Check sheet for the modelled part. Datum: model origin and axes. Units: mm. Round coordinates to 2 decimals unless told otherwise and drop trailing zeros. Write each loop counter-clockwise with the first axis right and the second up, starting at its lowest first coordinate (ties: lowest second). Pieces come first, ordered by that corner, then holes. Notation, with made-up numbers: (-25, -26.75) -> (-13, -26.75) arc R13 cw to (-13, -4.75) -> close; hole circle Ø5 at (53.25, 78.25). An arc over 180 degrees is marked (long way). Write item = value, one per line.
Solid Edge part; units mm, degrees
sketch "Sketch1" plane through (0, 0, 0) normal (0, 0, 1) x (1, 0, 0)
  line L0 (-36.25, 27.5) -> (36.25, 27.5)
  line L1 (36.25, 27.5) -> (36.25, -27.5)
  line L2 (36.25, -27.5) -> (-36.25, -27.5)
  line L3 (-36.25, -27.5) -> (-36.25, 27.5)
extrude "ExtrudedProtrusion_7" add sketch "Sketch1" along normal blind 4.8
sketch "Sketch2" plane through (0, 0, 4.8) normal (0, 0, 1) x (1, 0, 0)
  line L0 (-33.85, -15) -> (-31.45, -15)
  line L1 (-31.45, -11.9) -> (-31.45, 11.9)
  line L2 (-33.85, 15) -> (-31.45, 15)
  line L3 (-33.85, 15) -> (-33.85, -15)
  arc A0 (-31.45, -11.9) -> (-31.45, -15) centre (-31.45, -13.45) cw
  arc A1 (-31.45, 15) -> (-31.45, 11.9) centre (-31.45, 13.45) cw
  line L4 (31.45, -15) -> (33.85, -15)
  line L5 (33.85, -15) -> (33.85, 15)
  line L6 (33.85, 15) -> (31.45, 15)
  line L7 (31.45, 11.9) -> (31.45, -11.9)
  arc A2 (31.45, 11.9) -> (31.45, 15) centre (31.45, 13.45) cw
  arc A3 (31.45, -15) -> (31.45, -11.9) centre (31.45, -13.45) cw
extrude "ExtrudedCutout_13" cut sketch "Sketch2" against normal blind 2.4
sketch "Sketch3" plane through (0, 0, 4.8) normal (0, 0, 1) x (1, 0, 0)
  line L0 (-33.85, 11.9) -> (-33.85, -11.9)
  line L1 (-36.25, -15) -> (-33.85, -15)
  line L2 (-36.25, 15) -> (-36.25, -15)
  line L3 (-36.25, 15) -> (-33.85, 15)
  arc A0 (-33.85, 15) -> (-33.85, 11.9) centre (-33.85, 13.45) cw
  arc A1 (-33.85, -11.9) -> (-33.85, -15) centre (-33.85, -13.45) cw
  line L4 (36.25, 15) -> (33.85, 15)
  line L5 (36.25, -15) -> (36.25, 15)
  line L6 (33.85, -15) -> (36.25, -15)
  line L7 (33.85, 11.9) -> (33.85, -11.9)
  arc A2 (33.85, 11.9) -> (33.85, 15) centre (33.85, 13.45) cw
  arc A3 (33.85, -15) -> (33.85, -11.9) centre (33.85, -13.45) cw
extrude "ExtrudedCutout_14" cut sketch "Sketch3" against normal blind 4.8
properties material "Polycarbonate"
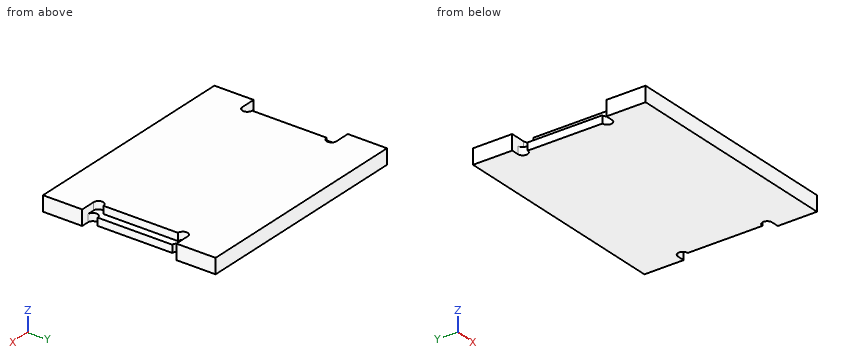
(1) Sectioned sample at B-B on z = 1.1. Enter the section's corners in (x, y).
Worked answers:
outline = (-36.25, -27.5) -> (36.25, -27.5) -> (36.25, -15) -> (33.85, -15) arc R1.55 cw to (33.85, -11.9) -> (33.85, 11.9) arc R1.55 cw to (33.85, 15) -> (36.25, 15) -> (36.25, 27.5) -> (-36.25, 27.5) -> (-36.25, 15) -> (-33.85, 15) arc R1.55 cw to (-33.85, 11.9) -> (-33.85, -11.9) arc R1.55 cw to (-33.85, -15) -> (-36.25, -15) -> close
(2) Material ranges on L1, parallel to Y at x = 33.5, z = 3.05; L2, parallel to Y at x = 33.5, z = 0.9; L3, parallel to Y at x = -32.5, z = 1.3, recorded low to high. Write a range as [from, to].
Worked answers:
L1 = [-27.5, -15], [15, 27.5]
L2 = [-27.5, -14.96], [-11.94, 11.94], [14.96, 27.5]
L3 = [-27.5, -14.21], [-12.69, 12.69], [14.21, 27.5]
(3) Go/stop test with flat-tipped pins: P1, Ø2.5, axis at y = -4.5, z = 1, coming from the +X side; P2, Ø1.9, axis at y = -4.5, z = 0.5, coming from the -X side; P3, Ø1.9, axis at y = 1, z = 4, coming from the +X side. Record where each tip stops, or that it passes through.
Worked answers:
P1 = 33.85
P2 = -33.85
P3 = 31.45
(4) Sectioned sample at A-A on y = -13.45. Enter the section's corners in (x, z).
Worked answers:
outline = (-32.3, 0) -> (32.3, 0) -> (32.3, 2.4) -> (29.9, 2.4) -> (29.9, 4.8) -> (-29.9, 4.8) -> (-29.9, 2.4) -> (-32.3, 2.4) -> close
